Autodesk Inventor part; units mm, degrees
ref_plane "Work Plane1" through (0, -12.4, 0) normal (0, 1, 0) x (-1, 0, 0)
ref_plane "YZ Plane" through (0, 0, 0) normal (1, 0, 0) x (0, 1, 0)
ref_plane "XY Plane" through (0, 0, 0) normal (0, 0, 1) x (1, 0, 0)
sketch "Sketch1" plane through (0, 0, 0) normal (0, 0, 1) x (1, 0, 0)
  circle A0 centre (0, 0) radius 12.4
  dimension "d0" = 24.8
extrude "Extrusion1" add sketch "Sketch1" against normal blind 56
sketch "Sketch2" plane through (0, 0, 0) normal (0, 0, 1) x (1, 0, 0)
  circle A0 centre (0, 0) radius 4
  dimension "d3" = 8
extrude "Extrusion2" add sketch "Sketch2" along normal blind 2.5
sketch "Sketch3" plane through (0, 0, 2.5) normal (0, 0, 1) x (1, 0, 0)
  circle A0 centre (0, 0) radius 2
  dimension "d6" = 4
extrude "Extrusion3" add sketch "Sketch3" along normal blind 9.5
sketch "Sketch4" plane through (0, 0, 0) normal (0, 0, 1) x (1, 0, 0)
  circle A0 centre (-8.5, 0) radius 1.5
  circle A1 centre (8.5, 0) radius 1.5
  circle A2 centre (0, 0) radius 2
  line L0 (-8.5, 0) -> (0, 0) construction
  line L1 (0, 0) -> (8.5, 0) construction
  dimension "d9" = 3
  dimension "d10" = 3
  dimension "d11" = 17
  dimension "d12" = 8.5
extrude "Extrusion4" cut sketch "Sketch4" against normal blind 8 contours A0 | A1
ref_plane "Work Plane1" through (0, -12.4, 0) normal (0, 1, 0) x (-1, 0, 0)
equation "\"d10\" = d9"
equation "\"d12\" = 0.5 * d11"
properties part number "motor"
Input: part model. Units: mm. Frame: model coordinates. A direction names the side the tool comes from. Round coordinates to 2 decimals unless told otherwise and drop trailing zeros. Loops run counter-clockwise (first coordinate to the right, second up) from the corner with the lowest first, then second, coordinate; pieces in that order, holes last. Notation, with made-up numbers: (80.5, 48) -> (122.5, 48) arc R12 ccw to (122.5, 56) -> close; hole circle Ø8 at (-8.75, -11). An arc over 180 degrees is marked (long way). Use one line per item in the form item = value. Start each with the question number.
Item 1: Section query A-A on x = 0. Return the cut outline in (y, z).
Item 2: Contact query for flat-ended pins moving along their axis: pin 1 Ø1.5 at (y, z) = (-9, -9.5) entering from -X; pin 2 Ø1.5 at (x, z) = (-7, -46) entering from -Y; pin 3 Ø7.5 at (x, y) = (5, 3) entering from +Z; pin 4 Ø8 at (y, z) = (2, -45.5) entering from +X. Output: stop coordinate, or through.
Item 3: Set-up query: faces 1 (the face through (7.3, -0.9, -3.9)), 2 (the face through (0, 0, -56)). Return all of +Z, -Z, +X, -X, +Y, -Y with unobstructed straight access to the full face (end or side cutting, diameter ignored); none if empty.
Item 4: Mould query, pull axis Y, two halves, no side actions, for faces 3 (the face through (-10, 0, -4)), 4 (the face through (5.72, -11, -27.61)), 5 (the face through (-2, -1, 2.5)). Classes: pulls with the +Y half, pulls with the -Y half, needs draft (parallel to the pull), parting line crosses it, or undercut.
Item 5: Section query B-B on y = 0. Return the cut outline in (x, z), then the cut area to 3 significant figures.
Item 6: Section query C-C on z = 7. Return the cut outline in (x, y).
Item 7: Material intervals for L1, parallel to Z at x = -0.5, y = -11; L2, parallel to Z at x = -9.75, y = -0.75; L3, parallel to Y at x = 0, z = -9.5, sorted ascending. Write a range as from..to.
Item 8: Section query D-D on z = -15.5. Return the cut outline in (x, y), then the cut area to 3 significant figures.
Ans:
q1.outline = (-12.4, -56) -> (12.4, -56) -> (12.4, 0) -> (4, 0) -> (4, 2.5) -> (2, 2.5) -> (2, 12) -> (-2, 12) -> (-2, 2.5) -> (-4, 2.5) -> (-4, 0) -> (-12.4, 0) -> close
q2.pin_1 = -9.26
q2.pin_2 = -10.71
q2.pin_3 = 2.5
q2.pin_4 = 12.4
q3.face_1 = +Z
q3.face_2 = -Z, +X, -X, +Y, -Y
q4.face_3 = undercut
q4.face_4 = parting line crosses it
q4.face_5 = needs draft
q5.outline = (-12.4, -56) -> (12.4, -56) -> (12.4, 0) -> (10, 0) -> (10, -8) -> (7, -8) -> (7, 0) -> (4, 0) -> (4, 2.5) -> (2, 2.5) -> (2, 12) -> (-2, 12) -> (-2, 2.5) -> (-4, 2.5) -> (-4, 0) -> (-7, 0) -> (-7, -8) -> (-10, -8) -> (-10, 0) -> (-12.4, 0) -> close
q5.area = 1,400 mm^2
q6.outline = circle Ø4 at (0, 0)
q7.L1 = -56..0
q7.L2 = -56..-8
q7.L3 = -12.4..12.4
q8.outline = circle Ø24.8 at (0, 0)
q8.area = 483 mm^2
